Here's how the part is built. I have some questions about the finished solid (model axes, mm). Face numbers are marked on the shaded views. A direction names the side the tool comes from. Coordinates: 2 decimals unless noted, no trailing zeros. Answer in a Markdown table with one row per item. Add a question column.
Item 1: On a 3-axis mill with a long thin cutter (end or side, diameter ignored), from which of +Z, -Z, +X, -X, +Y, -Y can I reach the whole of each face in a straight line? I mean the marked faces 1 and 2. Say none if no direction works.
Item 2: If I drill on line 1 along Y through (x, z) = (4, 1.5); line 2 along Y through (x, z) = (5, 3); line 3 along X through (y, z) = (8.25, 3.5), over which ranges is the centre line in solid material (lowest first)? Write a range as from..to.
Item 3: I want a section at A-A (z = 1.25). Count the separate pieces of the cut face and the enclosed holes in it, plus the area to 3 significant figures.
Item 4: Will these pins go through, and if not, where does the flat tip stop? pin 1 Ø0.6 at (x, z) = (2.5, 5.5) entering from -Y; pin 2 Ø2 at (y, z) = (10, 0.5) entering from -X.
Autodesk Inventor part; units mm, degrees
ref_plane "YZ Plane" through (0, 0, 0) normal (1, 0, 0) x (0, 1, 0)
ref_plane "XZ Plane" through (0, 0, 0) normal (0, 1, 0) x (-1, 0, 0)
ref_plane "XY Plane" through (0, 0, 0) normal (0, 0, 1) x (1, 0, 0)
sketch "Skizze5" plane through (0, 0, 0) normal (1, 0, 0) x (0, 1, 0)
  line L0 (0, 0) -> (0.5, 0)
  line L1 (0.5, 0) -> (4.9737, 0.486)
  line L2 (4.9737, 0.486) -> (11.4319, -0.2498)
  line L3 (11.4319, -0.2498) -> (11.9319, -0.2498)
  line L4 (11.9319, -0.2498) -> (11.9319, 5.2288)
  line L5 (11.9319, 5.2288) -> (4.9737, 6.0216)
  line L6 (0, 3.4663) -> (0, 0)
  line L7 (0, 3.4663) -> (4.9737, 4.0066)
  line L8 (4.9737, 8.0188) -> (4.9737, 2.9641) construction
  line L9 (4.9737, 6.0216) -> (4.9737, 4.0066)
  point P0 (0, 0)
  dimension "d21" = 0.5
  dimension "d22" = 6.2
  dimension "d23" = 6.5
  dimension "d24" = 4.5
  dimension "d25" = 6.5
  dimension "d26" = 5.5
  dimension "d27" = 3.5
extrude "Extrusion3" add sketch "Skizze5" along normal blind 8
sketch "Skizze6" plane through (8, 11.4319, -0.2498) normal (0, -0.1132032, -0.9935719) x (-1, 0, 0)
  circle A0 centre (4, -3.625) radius 2.425
  line L0 (4, 1.7492) -> (4, -8.8787)
  line L1 (-1.2914, -3.625) -> (9.5036, -3.625)
  line L2 (8, -0.1234) -> (8, -7.1266)
  line L3 (8, 0.4968) -> (0, 0.4968)
  point P0 (8, -11.3867)
  point P1 (8, -3.625)
  point P2 (4, 0.4968)
  dimension "d30" = 4.85
extrude "Extrusion4" cut sketch "Skizze6" against normal through all
sketch "Skizze7" plane through (8, 4.9737, 0.486) normal (0, 0.1079994, -0.994151) x (-1, 0, 0)
  line L0 (-0.408, -2.25) -> (9.5226, -2.25)
  line L1 (4, -0.248) -> (4, -7.2475)
  line L2 (8, -4.9971) -> (0, -4.9971)
  line L3 (8, -4.5) -> (8, 0)
  circle A0 centre (4, -2.25) radius 1.575
  point P0 (4, -4.9971)
  point P1 (8, -2.25)
  dimension "d33" = 3.15
extrude "Extrusion5" cut sketch "Skizze7" against normal through all
sketch "Skizze8" plane through (0, 11.4319, -0.2498) normal (0, 0, -1) x (-1, 0, 0)
  line L0 (-8, -6.4582) -> (-8, 0)
  line L1 (-8, -10.9319) -> (-8, -6.4582)
  line L2 (-8, -11.4319) -> (-8, -10.9319)
  line L3 (0, -11.4319) -> (-8, -11.4319)
  line L4 (0, -11.4319) -> (0, -10.9319)
  line L5 (0, -10.9319) -> (0, -6.4582)
  line L6 (0, -6.4582) -> (0, 0)
  line L7 (0, 0) -> (0, 0.5)
  line L8 (0, 0.5) -> (-8, 0.5)
  line L9 (-8, 0) -> (-8, 0.5)
extrude "Extrusion6" add sketch "Skizze8" against normal blind 0.75
sketch "Skizze9" plane through (0, 4.9737, 6.0216) normal (0, 0.1132032, 0.9935719) x (1, 0, 0)
  circle A0 centre (4, 3.5016) radius 2.425
  point P0 (0, -4.26)
extrude "Extrusion7" cut sketch "Skizze9" against normal through all
sketch "Skizze10" plane through (0, 0, 3.4663) normal (0, -0.1079994, 0.994151) x (1, 0, 0)
  circle A0 centre (4, 2.3727) radius 1.575
  point P0 (0, -0.3744)
extrude "Extrusion8" cut sketch "Skizze10" against normal through all
chamfer "Fase2" distance 0.5 angle 45 7 edges at (8, 5.9659, -0.2498) (4, 11.9319, -0.2498) (8, 11.9319, 2.4895) (0, 5.9659, -0.2498) (0, 11.9319, 2.4895) (8, 4.9737, 5.0141) (0, 4.9737, 5.0141)
chamfer "Fase3" distance 0.3 angle 45 2 edges at (6.425, 8.4528, 5.6252) (5.575, 2.3588, 3.7225)
properties part number "led_holder_v12"
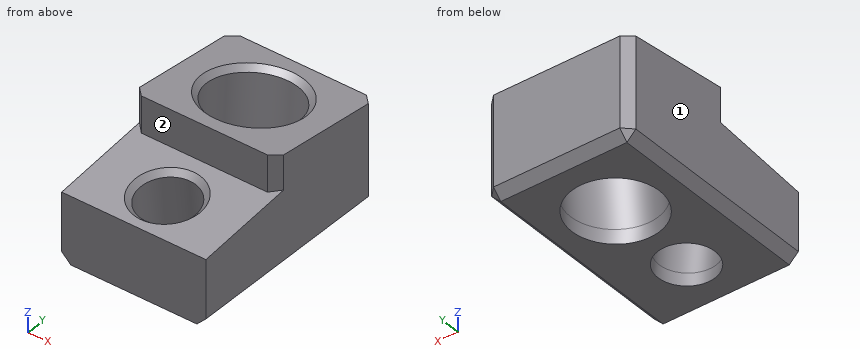
Values follow:
| question | item | result |
|---|---|---|
| 1 | face 1 | +Z, -Z, -X, +Y, -Y |
| 1 | face 2 | +Z, +X, -X, -Y |
| 2 | line 1 | y = 0..1.02, 4.18..5.54, 10.42..11.93 |
| 2 | line 2 | y = 0..1.21, 3.66..5.93, 10.38..11.93 |
| 2 | line 3 | x = 0..1.58, 6.42..8 |
| 3 | separate pieces | 1 |
| 3 | enclosed holes | 2 |
| 3 | area | 68.8 mm^2 |
| 4 | pin 1 | stops at y = 4.97 |
| 4 | pin 2 | stops at x = 0 |
